```python
from build123d import *

# Parameters (mm, degrees)
SKETCH1_W        = 50
SKETCH1_H        = 19
SKETCH1_R        = 2.5
BASE_PLATE_DEPTH = 2.5
SKETCH2_R        = 2.25
AXIS_DEPTH       = 15
FILLET1_R        = 2


with BuildPart() as part:
    # Sketch1 → Base Plate (new body)
    with BuildSketch(Plane(origin=(0, 0, 0), x_dir=(1, 0, 0), z_dir=(0, 1, 0))):
        with Locations((25, 9.5)):
            Rectangle(SKETCH1_W, SKETCH1_H)
        with Locations(Location((8.6, 9.5, 0), (0, 0, 270))):
            Circle(SKETCH1_R, mode=Mode.SUBTRACT)
    extrude(amount=BASE_PLATE_DEPTH)

    # Sketch2 → Axis (add)
    with BuildSketch(Plane(origin=(0, 2.5, 0), x_dir=(1, 0, 0), z_dir=(0, 1, 0))):
        with Locations(Location((40, 9.5, 0), (0, 0, 90))):
            Circle(SKETCH2_R)
    extrude(amount=AXIS_DEPTH)

    # Fillet1
    fillet1_edges = [part.edges().sort_by_distance(p)[0] for p in [
        (0, 1.25, -19),
        (50, 1.25, -19),
        (50, 1.25, 0),
        (0, 1.25, 0),
    ]]
    fillet(fillet1_edges, radius=FILLET1_R)


solid = part.part
```
Source: CAD feature listing. Evaluate the final solid. Frame: model axes, mm. A direction names the side the tool comes from. Give positions to 0.01 mm unless a question says otherwise; leave off trailing zeros. Loops run counter-clockwise (first coordinate to the right, second up) from the corner with the lowest first, then second, coordinate; pieces in that order, holes last. Notation, with made-up numbers: (-3, -17) -> (48, -17) arc R20 ccw to (48, 0) -> close; hole circle Ø1 at (-25, -21.5). An arc over 180 degrees is marked (long way). Put each result on its own line as item: value. Start each with the question number.
1) Material intervals for probe 1 along X at (y, z) = (1.2, -9.5); probe 2 along Z at (x, y) = (8.5, 2); probe 3 along Y at (x, z) = (33, -5.5), sorted ascending.
2) Cut plane D-D (y = 5.75). Return loops of the section in (x, z).
3) Contact query for flat-ended pins moving along their axis: P1, Ø1.5, axis at x = 14.5, z = -4.5, coming from the -Y side; P2, Ø10, axis at x = 38.5, z = -2, coming from the +Y side; P3, Ø1, axis at y = 5.5, z = -8.5, coming from the +X side; P4, Ø2, axis at x = 38.5, y = 13.5, coming from the -Z side. Output: stop coordinate, or through.
4) Cut plane C-C (x = 40). Return loops of the section in (y, z), then the cut area to 3 significant figures.
5) Cut plane A-A (z = -9.5). Return loops of the section in (x, y).
6) Cut plane B-B (x = 8.6). Return loops of the section in (y, z).
7) Draft query along Z for faces 3 (the face through (50, 1, -9)), 4 (the face through (25, 1, 0)), 5 (the face through (11.08, 1.23, -9.83)). Return one class per face: released by +Z, released by -Z, zero draft, split by the parting line, or undercut.
8) Reachability of faces 1 (the face through (40, 17.5, -9)), 2 (the face through (37.77, 9.9, -9.21)) from +Z, -Z, +X, -X, +Y, -Y: full face, straight path, thin tool, end or side. Return the list, or none.
Results are:
1. probe 1: x = 0 to 6.1, 11.1 to 50
1. probe 2: z = -19 to -12, -7 to 0
1. probe 3: y = 0 to 2.5
2. outline: circle Ø4.5 at (40, -9.5)
3. P1: stops at y = 0
3. P2: stops at y = 2.5
3. P3: stops at x = 42.19
3. P4: stops at z = -11.69
4. outline: (0, -19) -> (2.5, -19) -> (2.5, -11.75) -> (17.5, -11.75) -> (17.5, -7.25) -> (2.5, -7.25) -> (2.5, 0) -> (0, 0) -> close
4. area: 115 mm2
5. outline: (0, 0) -> (6.1, 0) -> (6.1, 2.5) -> (0, 2.5) -> close; (11.1, 0) -> (50, 0) -> (50, 2.5) -> (42.25, 2.5) -> (42.25, 17.5) -> (37.75, 17.5) -> (37.75, 2.5) -> (11.1, 2.5) -> close
6. outline: (0, -19) -> (2.5, -19) -> (2.5, -12) -> (0, -12) -> close; (0, -7) -> (2.5, -7) -> (2.5, 0) -> (0, 0) -> close
7. face 3: zero draft
7. face 4: released by +Z
7. face 5: undercut
8. face 1: +Z, -Z, +X, -X, +Y
8. face 2: +Y
